```python
from build123d import *

# Parameters (mm, degrees)
F0_R     = 6
F1_DEPTH = 25
F2_SIZE  = 80


with BuildPart() as f1:
    # F0 (on Right) → F1 (new body)
    with BuildSketch(Plane.YZ):
        Polygon((0, 740), (0, 0), (370, 0), (370, 310), (160, 310), (160, 510), (370, 510), (370, 704), (280, 704), (280, 560), (220, 560), (220, 704), (140, 704), (140, 740), align=None)
        with Locations((250, 205)):
            Circle(F0_R, mode=Mode.SUBTRACT)
    extrude(amount=F1_DEPTH)

    # F2
    f2_edges = [f1.edges().sort_by_distance(p)[0] for p in [
        (12.5, 0, 740),
    ]]
    chamfer(f2_edges, length=F2_SIZE)


solid = f1.part
```
For this review, take the finished solid that the model builds, in its own axes (mm). A direction names the side the tool comes from. Coordinates: 2 decimals unless noted, no trailing zeros. Write each loop counter-clockwise with the first axis right and the second up, starting at its lowest first coordinate (ties: lowest second). Pieces come first, ordered by that corner, then holes.
(1) Tool access review of faces 4 (the face through (12, 266, 310)), 5 (the face through (12, 280, 633)), 6 (the face through (12, 140, 722)): name each direction out of +Z, -Z, +X, -X, +Y, -Y from which nothing blocks a thin tool from reaching the whole face with its end or side.
(2) Add section B-B on x = 13. Give the boundary of the cut face in (y, z).
(3) Add section A-A on z = 583. Give the boundary of the cut face in (x, y).
(4) For pin 1 Ø7.5 at (x, z) = (15.5, 714) entering from +Y; pin 2 Ø8 at (x, y) = (3, 232.5) entering from +Z; pin 3 Ø12.5 at (x, y) = (10.5, 275) entering from +Z, all flat-tipped, find the tip position at first contact; note any pin that passes through.
(5) Add section C-C on y = 199. Give the boundary of the cut face in (x, z), then the cut area to 3 significant figures.
(6) Add section D-D on y = 48.5. Give the boundary of the cut face in (x, z).
(7) The part is to be moulded in two halves that separate along Z. For faces 1 (the face through (12, 0, 335)), 2 (the face through (12, 264, 510)), 3 (the face through (12, 250, 560)), say which applies: +Z half, -Z half, draft (parallel to the pull), parting line (faces both ways), or undercut.
(8) Wall thickness on probe 1 along Z at (x, y) = (9.25, 250); probe 2 along Z at (x, y) = (9, 319); probe 3 along Y at (x, z) = (6.75, 653.5): over which ranges is each line inside the solid? List them lowest first.
Answer sheet:
1. face 4: +X, -X, +Y
1. face 5: +Z, +X, -X
1. face 6: +Z, +X, -X, +Y
2. outline: (0, 0) - (370, 0) - (370, 310) - (160, 310) - (160, 510) - (370, 510) - (370, 704) - (280, 704) - (280, 560) - (220, 560) - (220, 704) - (140, 704) - (140, 740) - (80, 740) - (0, 660) - close; hole circle Ø12 at (250, 205)
3. outline: (0, 0) - (25, 0) - (25, 220) - (0, 220) - close; (0, 280) - (25, 280) - (25, 370) - (0, 370) - close
4. pin 1: stops at y = 140
4. pin 2: stops at z = 560
4. pin 3: stops at z = 704
5. outline: (0, 0) - (25, 0) - (25, 310) - (0, 310) - close; (0, 510) - (25, 510) - (25, 704) - (0, 704) - close
5. area: 12,600 mm2
6. outline: (0, 0) - (25, 0) - (25, 708.5) - (0, 708.5) - close
7. face 1: draft
7. face 2: undercut
7. face 3: +Z half
8. probe 1: z = 0 to 199, 211 to 310, 510 to 560
8. probe 2: z = 0 to 310, 510 to 704
8. probe 3: y = 0 to 220, 280 to 370
